Geometry check sheet. Reference: drawing and pictorial views, mm from the part's lowest x, y, z. Coordinates: 2 decimals unless noted, no trailing zeros. Order: outer loops, then holes, each group sorted by start corner. A loop starts at its lowest first (then second) coordinate and runs counter-clockwise, first axis right, second up. Notation, with made-up numbers: (-28.75, 26.5) -> (15.25, 26.5) arc R24 cw to (15.25, 45.5) -> close; hole circle Ø6 at (-28, 57.25). An arc over 180 degrees is marked (long way). Use CSV: the item, a comma, the result in double quotes. Start each with the question number.
1) Release check for a two-part mould opening along Y. For the marked faces 1, 2 and 3 record: released by +Y, released by -Y, zero draft, split by the parting line, or undercut.
2) Sectioned sample at A-A on z = 75. Record the boundary of the cut face in (x, y).
3) Sectioned sample at B-B on x = 25. Record the boundary of the cut face in (y, z).
4) Sectioned sample at D-D on y = 195. Record the boundary of the cut face in (x, z).
5) Scan lines: line 1 along X through (y, z) = (305.75, 75); line 2 along Y through (x, z) = (110.5, 139.5); line 3 along X through (y, z) = (306, 25). Record each from-to range of solid material in increasing order.
6) Go/stop test with flat-tipped pins: pin 1 (8 mm diameter, centred on x = 36.5, z = 24, fed in from -Y); pin 2 (19 mm diameter, centred on x = 75, z = 25, fed in from +Y). Record where each tip stops, or that it passes through.
7) Sectioned sample at C-C on z = 25. Record the boundary of the cut face in (x, y).
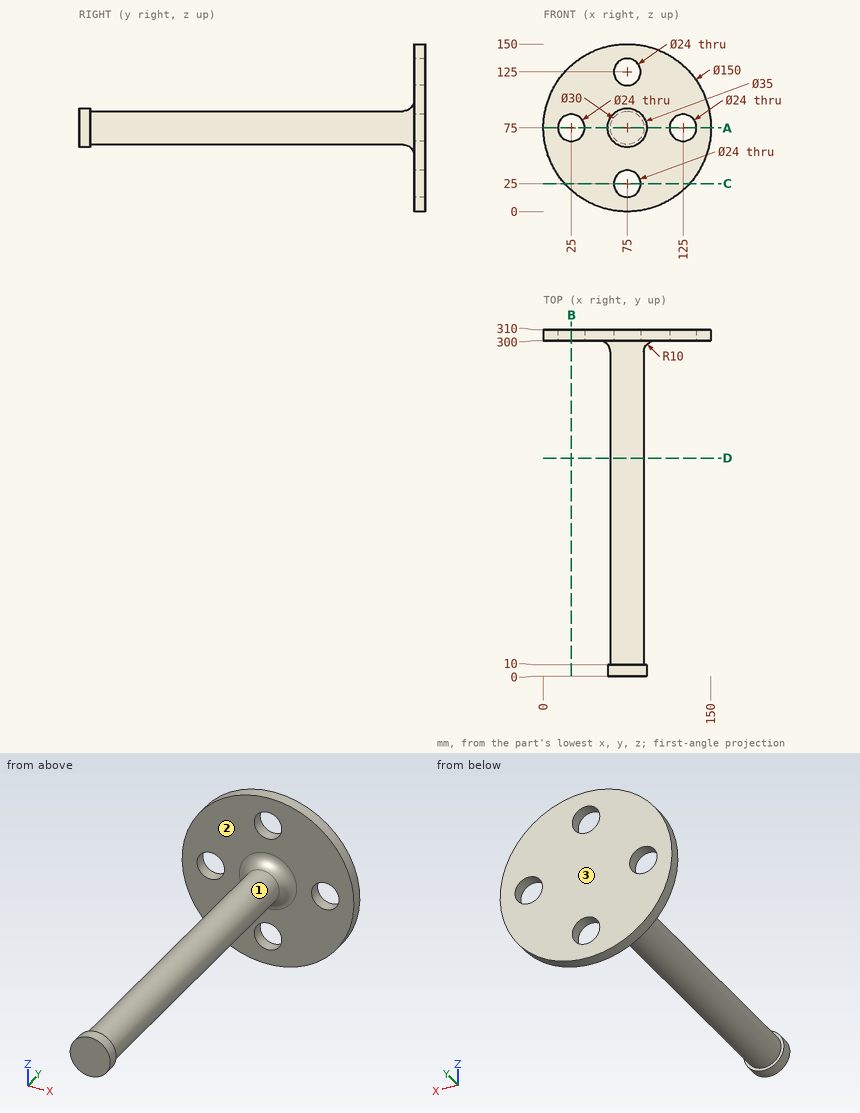
Answers follow:
1,face 1,"undercut"
1,face 2,"released by -Y"
1,face 3,"released by +Y"
2,outline,"(0, 300) -> (13, 300) -> (13, 310) -> (0, 310) -> close; (37, 300) -> (50, 300) arc R10 cw to (60, 290) -> (60, 10) -> (57.5, 10) -> (57.5, 0) -> (92.5, 0) -> (92.5, 10) -> (90, 10) -> (90, 290) arc R10 cw to (100, 300) -> (113, 300) -> (113, 310) -> (37, 310) -> close; (137, 300) -> (150, 300) -> (150, 310) -> (137, 310) -> close"
3,outline,"(300, 19.1) -> (310, 19.1) -> (310, 63) -> (300, 63) -> close; (300, 87) -> (310, 87) -> (310, 130.9) -> (300, 130.9) -> close"
4,outline,"circle Ø30 at (75, 75)"
5,line 1,"x = 0 to 13, 37 to 113, 137 to 150"
5,line 2,"y = 300 to 310"
5,line 3,"x = 19.1 to 63, 87 to 130.9"
6,pin 1,"stops at y = 300"
6,pin 2,"passes through"
7,outline,"(19.1, 300) -> (63, 300) -> (63, 310) -> (19.1, 310) -> close; (87, 300) -> (130.9, 300) -> (130.9, 310) -> (87, 310) -> close"
